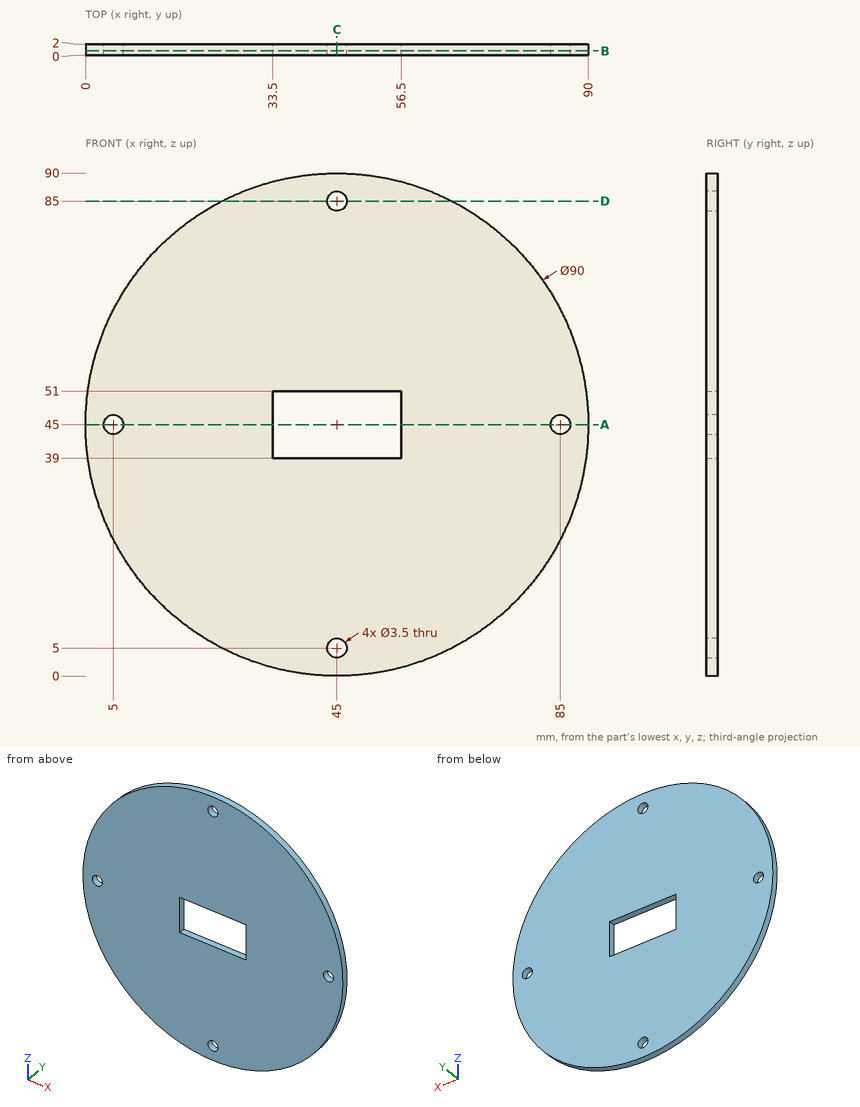
Geometry: see drawing. Coordinates: mm, zero at the bounding-box minimum. Give positions to 0.01 mm unless a question says otherwise; leave off trailing zeros. Loops run counter-clockwise (first coordinate to the right, second up) from the corner with the lowest first, then second, coordinate; pieces in that order, holes last. Notation, with made-up numbers: (65.25, 78.25) - (107.25, 78.25) arc R24 ccw to (107.25, 99.25) - close; hole circle Ø4 at (-1, 32.5). An arc over 180 degrees is marked (long way). Use CSV: the item, a comma, the result in double quotes. Start each with the question number.
1. Section D-D (z = 85). Output: boundary loops of the cut face in (x, y), then the cut area to 3 significant figures.
2. Ray query, L1, parallel to X at y = 0.75, z = 45; L2, parallel to X at y = 1.65, z = 85; L3, parallel to Z at x = 4, y = 1.15. Return the intervals inside material, ascending.
3. Pin query (flat end, axial travel): pin 1 (1 mm diameter, centred on x = 37, y = 1, fed in from -Z); pin 2 (3 mm diameter, centred on x = 45, z = 85, fed in from -Y) (3 decimals); pin 3 (1 mm diameter, centred on x = 41.5, y = 1, fed in from -Z); pin 4 (1 mm diameter, centred on y = 1, z = 43.5, fed in from +X). Return the tip coordinate at first contact, or that it passes through.
4. Section B-B (y = 0.75). Output: boundary loops of the cut face in (x, z), then the cut area to 3 significant figures.
5. Section C-C (x = 45). Output: boundary loops of the cut face in (y, z), then the cut area to 3 significant figures.
6. Section A-A (z = 45). Output: boundary loops of the cut face in (x, y).
Response:
1,outline,"(24.38, 0) - (43.25, 0) - (43.25, 2) - (24.38, 2) - close; (46.75, 0) - (65.62, 0) - (65.62, 2) - (46.75, 2) - close"
1,area,"75.5 mm²"
2,L1,"0 to 3.25, 6.75 to 33.5, 56.5 to 83.25, 86.75 to 90"
2,L2,"24.38 to 43.25, 46.75 to 65.62"
2,L3,"26.45 to 43.56, 46.44 to 63.55"
3,pin 1,"z = 0.63"
3,pin 2,"through"
3,pin 3,"z = 0.1"
3,pin 4,"x = 89.99"
4,outline,"circle Ø90 at (45, 45); hole circle Ø3.5 at (5, 45); hole (33.5, 39) - (56.5, 39) - (56.5, 51) - (33.5, 51) - close; hole circle Ø3.5 at (45, 5); hole circle Ø3.5 at (45, 85); hole circle Ø3.5 at (85, 45)"
4,area,"6,050 mm²"
5,outline,"(0, 0) - (2, 0) - (2, 3.25) - (0, 3.25) - close; (0, 6.75) - (2, 6.75) - (2, 39) - (0, 39) - close; (0, 51) - (2, 51) - (2, 83.25) - (0, 83.25) - close; (0, 86.75) - (2, 86.75) - (2, 90) - (0, 90) - close"
5,area,"142 mm²"
6,outline,"(0, 0) - (3.25, 0) - (3.25, 2) - (0, 2) - close; (6.75, 0) - (33.5, 0) - (33.5, 2) - (6.75, 2) - close; (56.5, 0) - (83.25, 0) - (83.25, 2) - (56.5, 2) - close; (86.75, 0) - (90, 0) - (90, 2) - (86.75, 2) - close"
